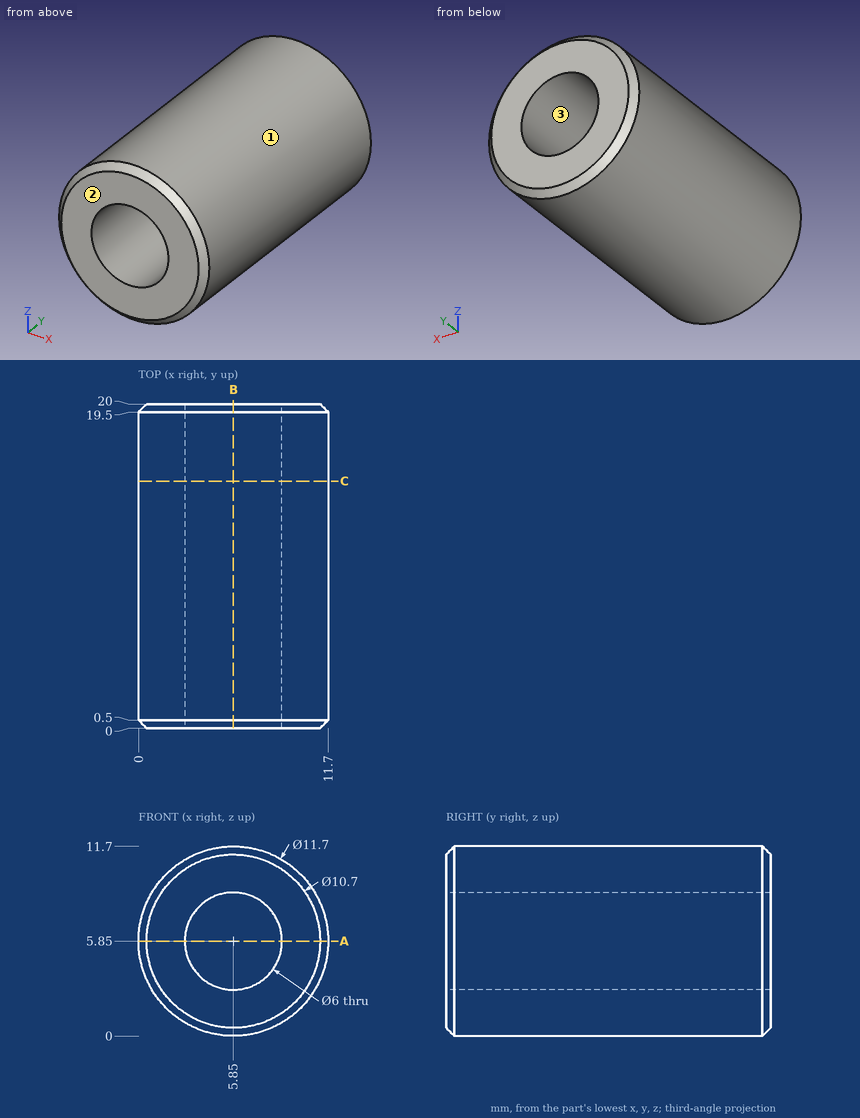
Can you work these out from the drawing? Everything is in mm from the part's minimum corner. Give positions to 0.01 mm unless a question says otherwise; leave off trailing zeros. Order: outer loops, then holes, each group sorted by start corner. A loop starts at its lowest first (then second) coordinate and runs counter-clockwise, first axis right, second up.
Item 1: I'm going to push flat-ended pins straight in: pin 1 (4 mm diameter, centred on y = 5.5, z = 3.5, fed in from +X); pin 2 (2 mm diameter, centred on y = 12, z = 10, fed in from -X); pin 3 (1 mm diameter, centred on y = 11.5, z = 1.5, fed in from +X); pin 4 (6 mm diameter, centred on x = 7, y = 2, fed in from -Z). Where does each tip first touch, or does it pass through?
Item 2: If we section it at B-B, the plane x = 5.85: Write out the boundary of the cut face in (y, z).
Item 3: If we section it at C-C, the plane y = 15.25: Write out the boundary of the cut face in (x, z), plus the area to 3 significant figures.
Item 4: I need wall thicknesses on line 1 (Z direction, x = 5.85, y = 13.5); line 2 (X direction, y = 3.75, z = 7.25); line 3 (X direction, y = 3.5, z = 7.75). Which ranges of each line are inside material? Lowest first, please.
Item 5: If we section it at A-A, the plane z = 5.85: Write out the boundary of the cut face in (x, y), plus the area to 4 significant figures.
Item 6: If we mould it in two halves opening along X, with no side actions, what happens to the marked faces 1, 2 and 3? For each: pulls with the +X half, pulls with the -X half, needs draft (parallel to the pull), parting line crosses it, or undercut.
Values:
1. pin 1: stops at x = 11.69
1. pin 2: stops at x = 0.92
1. pin 3: stops at x = 10.25
1. pin 4: stops at z = 0
2. outline: (0, 0.5) - (0.5, 0) - (19.5, 0) - (20, 0.5) - (20, 2.85) - (0, 2.85) - close; (0, 8.85) - (20, 8.85) - (20, 11.2) - (19.5, 11.7) - (0.5, 11.7) - (0, 11.2) - close
3. outline: circle Ø11.7 at (5.85, 5.85); hole circle Ø6 at (5.85, 5.85)
3. area: 79.2 mm2
4. line 1: z = 0 to 2.85, 8.85 to 11.7
4. line 2: x = 0.17 to 3.2, 8.5 to 11.53
4. line 3: x = 0.32 to 3.53, 8.17 to 11.38
5. outline: (0, 0.5) - (0.5, 0) - (2.85, 0) - (2.85, 20) - (0.5, 20) - (0, 19.5) - close; (8.85, 0) - (11.2, 0) - (11.7, 0.5) - (11.7, 19.5) - (11.2, 20) - (8.85, 20) - close
5. area: 113.5 mm2
6. face 1: parting line crosses it
6. face 2: needs draft
6. face 3: undercut
